CAD build for the part. Positions are in the model's coordinates, mm. A direction names the side the tool comes from. Coordinates: 2 decimals unless noted, no trailing zeros. Loops run counter-clockwise (first coordinate to the right, second up) from the corner with the lowest first, then second, coordinate; pieces in that order, holes last. Notation, with made-up numbers: (-23, 56) - (4, 56) arc R25 cw to (4, 83) - close; hole circle Ø3 at (41, 20). An arc over 180 degrees is marked (long way). Put each result on its own line as item: value.
```python
from build123d import *

# Parameters (mm, degrees)
F1_DEPTH = 6
F0_W     = 66
F0_H     = 121
F0_W_2   = 11.5
F0_H_2   = 1.5
F2_DEPTH = 3
F3_R     = 5
F4_DEPTH = 4


# Not quite as in the source:
# - a feature names something its author has since deleted; it is built from what else it names


with BuildPart() as f1:
    # F0 (on Top) → F1 (new body)
    with BuildSketch(Plane.XY):
        Polygon((30, -57.5), (30, 57.5), (28, 57.5), (28, -55.5), (-28, -55.5), (-28, 55.5), (14.5, 55.5), (14.5, 57.5), (-30, 57.5), (-30, -57.5), align=None)
    extrude(amount=F1_DEPTH)

    # F0 (on Top) → F2 (join)
    with BuildSketch(Plane.XY):
        Rectangle(F0_W, F0_H)
        Polygon((28, 57.5), (30, 57.5), (30, -57.5), (-30, -57.5), (-30, 57.5), (14.5, 57.5), (14.5, 55.5), (-28, 55.5), (-28, -55.5), (28, -55.5), align=None, mode=Mode.SUBTRACT)
        with Locations((21.25, 59)):
            Rectangle(F0_W_2, F0_H_2, mode=Mode.SUBTRACT)
    extrude(amount=F2_DEPTH)

    # F3
    f3_edges = [f1.edges().sort_by_distance(p)[0] for p in [
        (-33, 60.5, 1.5),
        (-33, -60.5, 1.5),
        (33, -60.5, 1.5),
        (33, 60.5, 1.5),
    ]]
    fillet(f3_edges, radius=F3_R)

    # F0 (on Top) → F4 (join)
    with BuildSketch(Plane.XY):
        with Locations((21.25, 59)):
            Rectangle(F0_W_2, F0_H_2)
    extrude(amount=F4_DEPTH)


solid = f1.part
```
Q1. Slice it at B-B, the plane y = 28.5. Give the cut face in (x, z).
Determined:
outline: (-33, 0) - (33, 0) - (33, 3) - (30, 3) - (30, 6) - (28, 6) - (28, 3) - (-28, 3) - (-28, 6) - (-30, 6) - (-30, 3) - (-33, 3) - close
Q2. Pin check, flat tips, straight feed: pin 1 Ø0.9 at (y, z) = (7.5, 4) entering from +X; pin 2 Ø0.9 at (x, z) = (6, 4) entering from +Y; pin 3 Ø0.8 at (x, z) = (24, 3.5) entering from +Y. Stop position of each tip, or through.
Determined:
pin 1: x = 30
pin 2: y = 57.5
pin 3: y = 59.75
Q3. Tool access for faces 4 (the flat face through (0, -57.5, 4)), 5 (the flat face through (-30, 1, 4)), 6 (the flat face through (-7, 57.5, 4)), 7 (the flat face through (30, -1, 4)), 8 (the flat face through (-7, 55.5, 4)): list every direction of +Z, -Z, +X, -X, +Y, -Y with a clear straight run to the whole face (end or side of a thin tool).
Determined:
face 4: +Z, +X, -X, -Y
face 5: +Z, -X, +Y, -Y
face 6: +Z, +X, -X, +Y
face 7: +Z, +X, +Y, -Y
face 8: +Z
Q4. Slice it at A-A, the plane x = -18. Give the cut face in (y, z), then the cut area to 3 significant figures.
Determined:
outline: (-60.5, 0) - (60.5, 0) - (60.5, 3) - (57.5, 3) - (57.5, 6) - (55.5, 6) - (55.5, 3) - (-55.5, 3) - (-55.5, 6) - (-57.5, 6) - (-57.5, 3) - (-60.5, 3) - close
area: 375 mm2
Q5. Mould opens along Y. For faces 1 (the cylindrical face through (31.5, -59.07, 1.52)), 2 (the flat face through (0, -55.5, 4)), 3 (the cylindrical face through (-31.57, 59, 1.52)) say: +Y half, -Y half, draft (parallel to the pull), parting line (faces both ways), or undercut.
Determined:
face 1: -Y half
face 2: undercut
face 3: +Y half
Q6. Wall check: L1, parallel to Y at x = 3, z = 5.6; L2, parallel to X at y = 35, z = 4.2; L3, parallel to Y at x = 29, z = 5.6. Give the ranges that are in metal, low to high. Write a range as from..to.
Determined:
L1: -57.5..-55.5, 55.5..57.5
L2: -30..-28, 28..30
L3: -57.5..57.5
